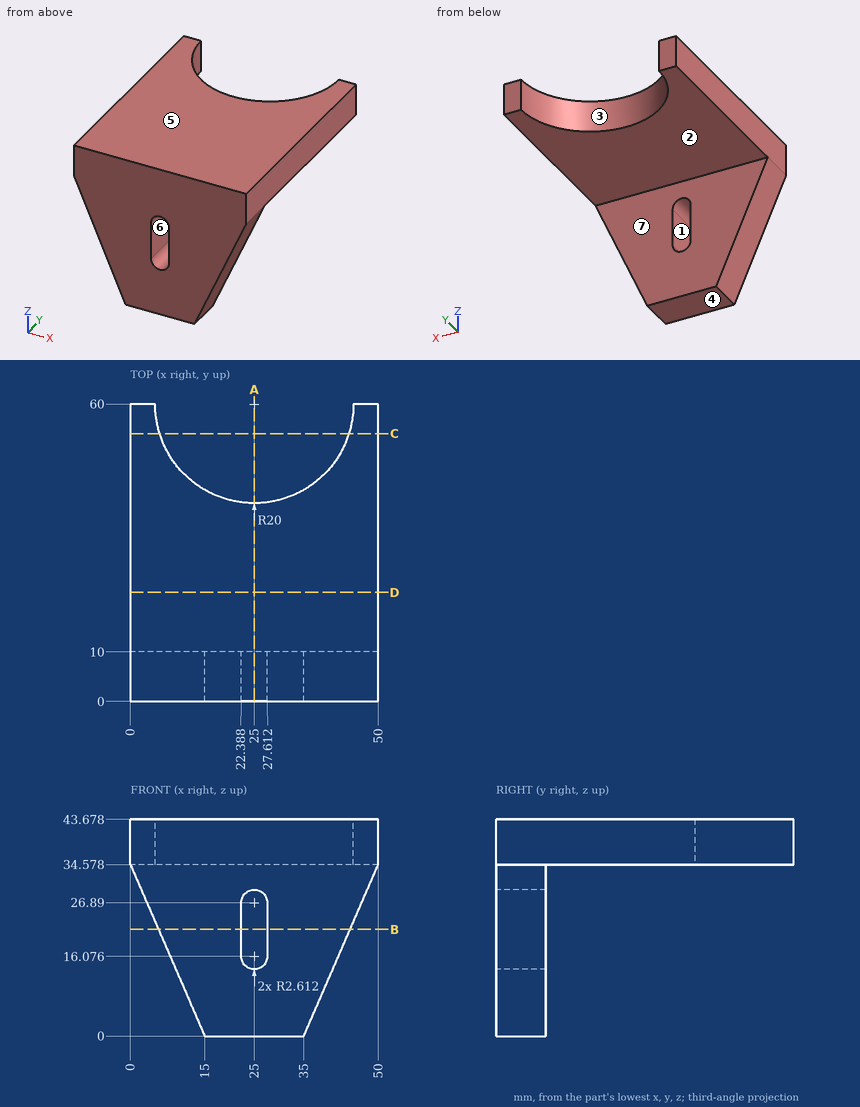
Can you work these out from the drawing? Everything is in mm from the part's minimum corner. A direction names the side the tool comes from. Round coordinates to 2 decimals unless told otherwise and drop trailing zeros. Loops run counter-clockwise (first coordinate to the right, second up) from the corner with the lowest first, then second, coordinate; pieces in that order, holes last. Notation, with made-up numbers: (-9.75, 31.5) - (2.25, 31.5) arc R29 ccw to (2.25, 51.5) - close; hole circle Ø11 at (-34, -1). An arc over 180 degrees is marked (long way). Answer in a Markdown table with one row per item. Add a question column.
Q1. I want a section at D-D on y = 22. List the corners of the cut face in (x, z) for me.
Q2. I need wall thicknesses on L1, parallel to Z at x = 3, y = 38; L2, parallel to Y at x = 37, z = 30; L3, parallel to Z at x = 12, y = 6 (1 decimal). Which ranges of each line are inside material? Lowest first, please.
Q3. Which directions (+Z, -Z, +X, -X, +Y, -Y) give clear straight access to the entire face, cutting with the end or side of a thin tool? Please do the marked faces 1, 2 and 3.
Q4. I want a section at C-C on y = 54. List the corners of the cut face in (x, z) for me.
Q5. I want a section at A-A on x = 25. List the corners of the cut face in (y, z) for me.
Q6. We'd pull the mould along Z, two halves only. Please class the marked faces 4, 5, 6 and 7: pulls with the +Z half, pulls with the -Z half, needs draft (parallel to the pull), parting line crosses it, or undercut.
Q7. I want a section at B-B on z = 21.5. List the corners of the cut face in (x, y) for me, and give its area (3 significant figures).
Q8. For pin 1 Ø8 at (x, z) = (29, 15) entering from -Y; pin 2 Ø6 at (x, z) = (40, 25) entering from +Y; pin 3 Ø5 at (y, z) = (4.5, 22.5) entering from +X (1 decimal); pin 4 Ø11 at (y, z) = (3, 19) entering from -X, each with a flat end and sliding along its axis, tell me the tip position at first contact or that it passes through.
A:
| question | item | result |
|---|---|---|
| 1 | outline | (0, 34.58) - (50, 34.58) - (50, 43.68) - (0, 43.68) - close |
| 2 | L1 | 34.58 to 43.68 |
| 2 | L2 | 0 to 10 |
| 2 | L3 | 6.9 to 43.7 |
| 3 | face 1 | +Y, -Y |
| 3 | face 2 | -Z, +X, -X, +Y |
| 3 | face 3 | +Z, -Z, +Y |
| 4 | outline | (0, 34.58) - (5.92, 34.58) - (5.92, 43.68) - (0, 43.68) - close; (44.08, 34.58) - (50, 34.58) - (50, 43.68) - (44.08, 43.68) - close |
| 5 | outline | (0, 0) - (10, 0) - (10, 13.46) - (0, 13.46) - close; (0, 29.5) - (10, 29.5) - (10, 34.58) - (40, 34.58) - (40, 43.68) - (0, 43.68) - close |
| 6 | face 4 | pulls with the -Z half |
| 6 | face 5 | pulls with the +Z half |
| 6 | face 6 | undercut |
| 6 | face 7 | needs draft |
| 7 | outline | (5.67, 0) - (22.39, 0) - (22.39, 10) - (5.67, 10) - close; (27.61, 0) - (44.33, 0) - (44.33, 10) - (27.61, 10) - close |
| 7 | area | 334 mm^2 |
| 8 | pin 1 | y = 0 |
| 8 | pin 2 | y = 10 |
| 8 | pin 3 | x = 45.8 |
| 8 | pin 4 | x = 4.37 |
